The listing builds one solid part. Answer for the finished solid, in the listing's coordinates (mm). A direction names the side the tool comes from. Coordinates: 2 decimals unless noted, no trailing zeros. Write each question's results on one line, items separated by ' | '. Start each with the question number.
(1) For faces 3 (the cylindrical face through (62.123, 0.093, 1.268)), 4 (the flat face through (28, -7.32, 4)), 5 (the flat face through (27, 27.5, 1)), determine the directions among +Z, -Z, +X, -X, +Y, -Y from which every point of the face is accessible in a straight line to the end or side of a thin tool.
(2) Given pin 1 Ø12 at (x, y) = (70.5, 6) entering from -Z; pin 2 Ø4 at (y, z) = (5, 5) entering from +X; pin 3 Ø1 at (x, y) = (-1.5, -2) entering from -Z, each flat-ended and moving along its own axis, determine where each tip first touches the part or whether it passes through.
(3) Consider line 1 (X direction, y = -9, z = 0.5); line 2 (Z direction, x = 103, y = -7.5); line 3 (X direction, y = 13, z = 1). Determine where each line is inside the solid, lowest interval first. Write a range as from..to.
(4) Find section A-A on z = 1.25. State how many separate pieces and enclosed holes the cut face has, then the cut area to 3 significant figures.
(5) Determine the mould class of faces 1 (the flat face through (54, 0, 7)), 2 (the flat face through (82, 16.922, 4)) for opening direction X: released by +X, released by -X, zero draft, split by the parting line, or undercut.
from build123d import *
from OCP.BRepFilletAPI import BRepFilletAPI_MakeChamfer

# Parameters (mm, degrees)
BOSS_EXTRUDE1_DEPTH = 7
CHAMFER1_SIZE       = 4
CHAMFER1_SIZE2      = 6.92820323
SKETCH3_R           = 8.5
CUT_EXTRUDE2_DEPTH  = 4
CUT_EXTRUDE3_DEPTH  = 3.5
SKETCH5_3_R         = 2.125
CUT_EXTRUDE4_DEPTH  = 141.295224438
CHAMFER2_SIZE       = 0.5
CHAMFER2_SIZE2      = 1.37373871
BOSS_EXTRUDE2_START = 0.5
SKETCH7_R           = 9.5
SKETCH7_R_2         = 8.5
BOSS_EXTRUDE2_DEPTH = 0.5


with BuildPart() as part:
    # Sketch1 → Boss-Extrude1 (new body)
    with BuildSketch(Plane.XY):
        with BuildLine():
            Line((52.546312184, 27.5), (0, 27.5))
            ThreePointArc((0, 27.5), (-27.5, 0), (0, -27.5))
            ThreePointArc((0, -27.5), (20.821970152, -25.821648832), (41.106300643, -20.829931677))
            ThreePointArc((41.106300643, -20.829931677), (78.372680186, -13.821988034), (116.152736046, -17.071864575))
            ThreePointArc((116.152736046, -17.071864575), (136.920766347, -4.465161388), (125.077159298, 16.747311828))
            ThreePointArc((125.077159298, 16.747311828), (89.208090939, 24.797217895), (52.546312184, 27.5))
        make_face()
    extrude(amount=BOSS_EXTRUDE1_DEPTH)

    # Chamfer1: one chamfer whose edges measure the first distance from different faces: ONE call of the kernel's chamfer builder (chamfer() names one face for all edges)
    chamfer1_edges_1 = [part.edges().sort_by_distance(p)[0] for p in [
        (78.372680186, -13.821988034, 7),
    ]]
    chamfer1_side_1 = [part.faces().sort_by_distance(p)[0] for p in [
        (78.372680186, -13.821988034, 3.5),
    ]]
    chamfer1_edges_2 = [part.edges().sort_by_distance(p)[0] for p in [
        (136.920766347, -4.465161388, 7),
    ]]
    chamfer1_side_2 = [part.faces().sort_by_distance(p)[0] for p in [
        (136.920766347, -4.465161388, 3.5),
    ]]
    chamfer1_edges_3 = [part.edges().sort_by_distance(p)[0] for p in [
        (89.208090939, 24.797217895, 7),
    ]]
    chamfer1_side_3 = [part.faces().sort_by_distance(p)[0] for p in [
        (89.208090939, 24.797217895, 3.5),
    ]]
    chamfer1_edges_4 = [part.edges().sort_by_distance(p)[0] for p in [
        (26.273156092, 27.5, 7),
    ]]
    chamfer1_side_4 = [part.faces().sort_by_distance(p)[0] for p in [
        (26.273156092, 27.5, 3.5),
    ]]
    chamfer1_edges_5 = [part.edges().sort_by_distance(p)[0] for p in [
        (-27.5, 0, 7),
    ]]
    chamfer1_side_5 = [part.faces().sort_by_distance(p)[0] for p in [
        (-27.5, 0, 3.5),
    ]]
    chamfer1_edges_6 = [part.edges().sort_by_distance(p)[0] for p in [
        (20.821970152, -25.821648832, 7),
    ]]
    chamfer1_side_6 = [part.faces().sort_by_distance(p)[0] for p in [
        (20.821970152, -25.821648832, 3.5),
    ]]
    chamfer1 = BRepFilletAPI_MakeChamfer(part.part.solid().wrapped)
    for e in chamfer1_edges_1:
        chamfer1.Add(CHAMFER1_SIZE, CHAMFER1_SIZE2, e.wrapped, chamfer1_side_1[0].wrapped)  # the first distance lies on this face
    for e in chamfer1_edges_2:
        chamfer1.Add(CHAMFER1_SIZE, CHAMFER1_SIZE2, e.wrapped, chamfer1_side_2[0].wrapped)  # the first distance lies on this face
    for e in chamfer1_edges_3:
        chamfer1.Add(CHAMFER1_SIZE, CHAMFER1_SIZE2, e.wrapped, chamfer1_side_3[0].wrapped)  # the first distance lies on this face
    for e in chamfer1_edges_4:
        chamfer1.Add(CHAMFER1_SIZE, CHAMFER1_SIZE2, e.wrapped, chamfer1_side_4[0].wrapped)  # the first distance lies on this face
    for e in chamfer1_edges_5:
        chamfer1.Add(CHAMFER1_SIZE, CHAMFER1_SIZE2, e.wrapped, chamfer1_side_5[0].wrapped)  # the first distance lies on this face
    for e in chamfer1_edges_6:
        chamfer1.Add(CHAMFER1_SIZE, CHAMFER1_SIZE2, e.wrapped, chamfer1_side_6[0].wrapped)  # the first distance lies on this face
    add(Compound.cast(chamfer1.Shape()), mode=Mode.REPLACE)

    # Sketch3 → Cut-Extrude2 (cut)
    with BuildSketch(Plane(origin=(0, 0, 0), x_dir=(-1, 0, 0), z_dir=(0, 0, -1))):
        Circle(SKETCH3_R)
        with Locations((-120, 0)):
            Circle(SKETCH3_R)
    extrude(amount=-CUT_EXTRUDE2_DEPTH, mode=Mode.SUBTRACT)

    # Sketch5 → Cut-Extrude3 (cut)
    with BuildSketch(Plane(origin=(0, 0, 2.5), x_dir=(-1, 0, 0), z_dir=(0, 0, -1))):
        with BuildLine():
            Line((-86.046403676, 16.921929528), (-88.139298402, 13.296929528))
            Line((-88.139298402, 13.296929528), (-86.046403676, 9.671929528))
            Line((-86.046403676, 9.671929528), (-78.548867374, 9.671929528))
            ThreePointArc((-78.548867374, 9.671929528), (-67.767719499, 13.296929528), (-78.548867374, 16.921929528))
            Line((-78.548867374, 16.921929528), (-86.046403676, 16.921929528))
        make_face()
        with BuildLine():
            Line((-62.092894726, -3.625), (-54.595358423, -3.625))
            ThreePointArc((-54.595358423, -3.625), (-43.814210548, 0), (-54.595358423, 3.625))
            Line((-54.595358423, 3.625), (-62.092894726, 3.625))
            Line((-62.092894726, 3.625), (-64.185789452, 0))
            Line((-64.185789452, 0), (-62.092894726, -3.625))
        make_face()
        with BuildLine():
            Line((-32.163058591, -14.569644586), (-24.665522288, -14.569644586))
            ThreePointArc((-24.665522288, -14.569644586), (-13.884374414, -10.944644586), (-24.665522288, -7.319644586))
            Line((-24.665522288, -7.319644586), (-32.163058591, -7.319644586))
            Line((-32.163058591, -7.319644586), (-34.255953317, -10.944644586))
            Line((-34.255953317, -10.944644586), (-32.163058591, -14.569644586))
        make_face()
    extrude(amount=-CUT_EXTRUDE3_DEPTH, mode=Mode.SUBTRACT)

    # Sketch5_3 → Cut-Extrude4 (cut, through all)
    with BuildSketch(Plane(origin=(0, 0, 2.5), x_dir=(-1, 0, 0), z_dir=(0, 0, -1))):
        with BuildLine():
            ThreePointArc((-78.548867374, 9.671929528), (-67.767719499, 13.296929528), (-78.548867374, 16.921929528))
            ThreePointArc((-78.548867374, 16.921929528), (-79.767719499, 13.296929528), (-78.548867374, 9.671929528))
        make_face()
        with BuildLine():
            ThreePointArc((-54.595358423, 3.625), (-55.814210548, 0), (-54.595358423, -3.625))
            ThreePointArc((-54.595358423, -3.625), (-43.814210548, 0), (-54.595358423, 3.625))
        make_face()
        with BuildLine():
            ThreePointArc((-24.665522288, -7.319644586), (-25.884374414, -10.944644586), (-24.665522288, -14.569644586))
            ThreePointArc((-24.665522288, -14.569644586), (-13.884374414, -10.944644586), (-24.665522288, -7.319644586))
        make_face()
        with Locations((-83.953508951, 13.296929528)):
            Circle(SKETCH5_3_R)
        with Locations((-60, 0)):
            Circle(SKETCH5_3_R)
        with Locations((-30.070163865, -10.944644586)):
            Circle(SKETCH5_3_R)
    extrude(amount=CUT_EXTRUDE4_DEPTH, mode=Mode.SUBTRACT)

    # Chamfer2: one chamfer whose edges measure the first distance from different faces: ONE call of the kernel's chamfer builder (chamfer() names one face for all edges)
    chamfer2_edges_1 = [part.edges().sort_by_distance(p)[0] for p in [
        (13.884374414, -10.944644586, 6),
    ]]
    chamfer2_side_1 = [part.faces().sort_by_distance(p)[0] for p in [
        (15.103226539, -14.569644586, 3),
    ]]
    chamfer2_edges_2 = [part.edges().sort_by_distance(p)[0] for p in [
        (43.814210548, 0, 6),
    ]]
    chamfer2_side_2 = [part.faces().sort_by_distance(p)[0] for p in [
        (45.033062674, -3.625, 3),
    ]]
    chamfer2_edges_3 = [part.edges().sort_by_distance(p)[0] for p in [
        (67.767719499, 13.296929528, 6),
    ]]
    chamfer2_side_3 = [part.faces().sort_by_distance(p)[0] for p in [
        (68.986571624, 9.671929528, 3),
    ]]
    chamfer2 = BRepFilletAPI_MakeChamfer(part.part.solid().wrapped)
    for e in chamfer2_edges_1:
        chamfer2.Add(CHAMFER2_SIZE, CHAMFER2_SIZE2, e.wrapped, chamfer2_side_1[0].wrapped)  # the first distance lies on this face
    for e in chamfer2_edges_2:
        chamfer2.Add(CHAMFER2_SIZE, CHAMFER2_SIZE2, e.wrapped, chamfer2_side_2[0].wrapped)  # the first distance lies on this face
    for e in chamfer2_edges_3:
        chamfer2.Add(CHAMFER2_SIZE, CHAMFER2_SIZE2, e.wrapped, chamfer2_side_3[0].wrapped)  # the first distance lies on this face
    add(Compound.cast(chamfer2.Shape()), mode=Mode.REPLACE)

    # Sketch7 → Boss-Extrude2 (add)
    # profile 1 of 2: a face of its own
    with BuildSketch(Plane(origin=(0, 0, 0), x_dir=(-1, 0, 0), z_dir=(0, 0, -1)).offset(BOSS_EXTRUDE2_START)):
        with Locations(Location((0, 0, 0), (0, 0, 180))):
            Circle(SKETCH7_R)
        Circle(SKETCH7_R_2, mode=Mode.SUBTRACT)
    # profile 2 of 2: a face of its own
    with BuildSketch(Plane(origin=(0, 0, 0), x_dir=(-1, 0, 0), z_dir=(0, 0, -1)).offset(BOSS_EXTRUDE2_START)):
        with Locations(Location((-120, 0, 0), (0, 0, 180))):
            Circle(SKETCH7_R)
        with Locations((-120, 0)):
            Circle(SKETCH7_R_2, mode=Mode.SUBTRACT)
    extrude(amount=-BOSS_EXTRUDE2_DEPTH)


solid = part.part
Values:
1) face 3: -Z | face 4: none | face 5: +Z, -Z, +X, -X, +Y
2) pin 1: stops at z = 0 | pin 2: stops at x = 136.82 | pin 3: stops at z = 4
3) line 1: x = -25.99..14.21, 25.56..29.21, 30.93..135.01 | line 2: z = 0..7 | line 3: x = -24.23..67.78, 79.76..81.85, 86.06..131.72
4) separate pieces: 1 | enclosed holes: 8 | area: 6,200 mm²
5) face 1: zero draft | face 2: undercut
